Here's how the part is built. I have some questions about the finished solid (model axes, mm). Coordinates: 2 decimals unless noted, no trailing zeros. Write each loop counter-clockwise with the first axis right and the second up, starting at its lowest first coordinate (ties: lowest second). Pieces come first, ordered by that corner, then holes.
Item 1: I'm going to push flat-ended pins straight in: P1, Ø3, axis at x = 210, y = 126.5, coming from the -Z side; P2, Ø3.5, axis at x = 6.35, y = 76.2, coming from the -Z side; P3, Ø5, axis at x = 125.5, z = 2.5, coming from the +Y side. Where does each tip first touch, or does it pass through?
Item 2: Please list where these lines run through material, in increasing order: line 1 (X direction, y = 203.2, z = 5); line 2 (X direction, y = 321, z = 3.5); line 3 (Y direction, x = 164.5, z = 7).
Item 3: I want a section at A-A (y = 38.5). Please give me the cut outline in (x, z).
Item 4: I want a section at B-B (z = 7.5). Count the separate pieces of the cut face and the enclosed holes in it, and give its area (3 significant figures).
Item 5: I want a section at C-C (x = 169). Please give me the cut outline in (y, z).
from build123d import *

# Parameters (mm, degrees)
SKETCH1_W           = 304.8
SKETCH1_H           = 355.6
BOSS_EXTRUDE1_DEPTH = 12.7
SKETCH2_W           = 228.6
SKETCH2_H           = 88.9
CUT_EXTRUDE1_DEPTH  = 469.525015341
SKETCH3_R           = 2.159
CUT_EXTRUDE2_DEPTH  = 469.525015341


with BuildPart() as part:
    # Sketch1 → Boss-Extrude1 (new body)
    with BuildSketch(Plane.XY):
        with Locations((152.4, 177.8)):
            Rectangle(SKETCH1_W, SKETCH1_H)
    extrude(amount=BOSS_EXTRUDE1_DEPTH)

    # Sketch2 → Cut-Extrude1 (cut, through all)
    with BuildSketch(Plane.XY.offset(12.7)):
        with Locations((152.4, 44.45)):
            Rectangle(SKETCH2_W, SKETCH2_H)
        with Locations((152.4, 311.15)):
            Rectangle(SKETCH2_W, SKETCH2_H)
    extrude(amount=-CUT_EXTRUDE1_DEPTH, mode=Mode.SUBTRACT)

    # Sketch3 → Cut-Extrude2 (cut, through all)
    with BuildSketch(Plane.XY.offset(12.7)):
        with Locations((6.35, 330.2)):
            Circle(SKETCH3_R)
        with Locations((6.35, 279.4)):
            Circle(SKETCH3_R)
        with Locations(Location((6.35, 76.2, 0), (0, 0, 180))):
            Circle(SKETCH3_R)
        with Locations(Location((6.35, 25.4, 0), (0, 0, 180))):
            Circle(SKETCH3_R)
        with Locations((298.45, 25.4)):
            Circle(SKETCH3_R)
        with Locations((298.45, 76.2)):
            Circle(SKETCH3_R)
        with Locations(Location((298.45, 279.4, 0), (0, 0, 180))):
            Circle(SKETCH3_R)
        with Locations(Location((298.45, 330.2, 0), (0, 0, 180))):
            Circle(SKETCH3_R)
        with Locations(Location((6.35, 203.2, 0), (0, 0, 180))):
            Circle(SKETCH3_R)
        with Locations(Location((6.35, 152.4, 0), (0, 0, 180))):
            Circle(SKETCH3_R)
        with Locations((298.45, 152.4)):
            Circle(SKETCH3_R)
        with Locations((298.45, 203.2)):
            Circle(SKETCH3_R)
    extrude(amount=-CUT_EXTRUDE2_DEPTH, mode=Mode.SUBTRACT)


solid = part.part
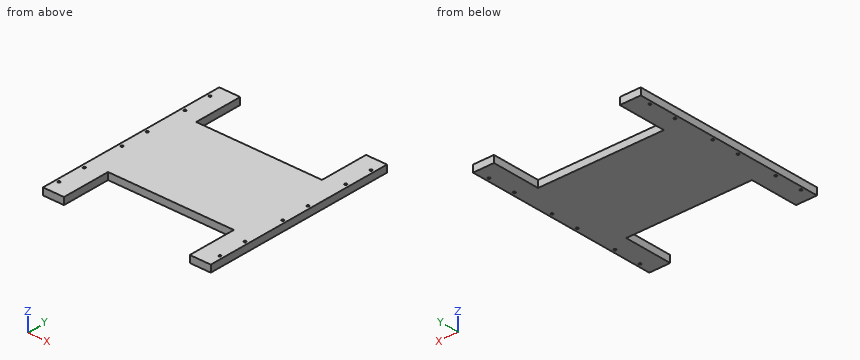
Answer:
1. P1: stops at z = 0
1. P2: passes through
1. P3: stops at y = 266.7
2. line 1: x = 0 to 4.19, 8.51 to 296.29, 300.61 to 304.8
2. line 2: x = 0 to 38.1, 266.7 to 304.8
2. line 3: y = 88.9 to 266.7
3. outline: (0, 0) - (38.1, 0) - (38.1, 12.7) - (0, 12.7) - close; (266.7, 0) - (304.8, 0) - (304.8, 12.7) - (266.7, 12.7) - close
4. separate pieces: 1
4. enclosed holes: 12
4. area: 67,600 mm2
5. outline: (88.9, 0) - (266.7, 0) - (266.7, 12.7) - (88.9, 12.7) - close
